from build123d import *

# Parameters (mm, degrees)
SKETCH_1_W          = 20
SKETCH_1_H          = 20
EXTRUDE_1_DEPTH     = 145
SKETCH_2_R          = 2.75
CUT_EXTRUDE_1_DEPTH = 20
SKETCH_4_R          = 1.5
CUT_EXTRUDE_4_DEPTH = 20


with BuildPart() as part:
    # 草图1 → 凸台-拉伸1 (new body)
    with BuildSketch(Plane.XY):
        Rectangle(SKETCH_1_W, SKETCH_1_H)
    extrude(amount=EXTRUDE_1_DEPTH)

    # 草图2 → 切除-拉伸1 (cut)
    with BuildSketch(Plane(origin=(10, 0, 0), x_dir=(0, 0, -1), z_dir=(1, 0, 0))):
        with Locations((-136, 3)):
            Circle(SKETCH_2_R)
        with Locations((-104, 3)):
            Circle(SKETCH_2_R)
        with Locations((-9, 3)):
            Circle(SKETCH_2_R)
        with Locations((-41, 3)):
            Circle(SKETCH_2_R)
    extrude(amount=-CUT_EXTRUDE_1_DEPTH, mode=Mode.SUBTRACT)

    # 草图4 → 切除-拉伸4 (cut)
    with BuildSketch(Plane(origin=(0, 10, 0), x_dir=(1, 0, 0), z_dir=(0, 1, 0))):
        with Locations(Location((-4.85, -24.606973042, 0), (0, 0, 270))):
            Circle(SKETCH_4_R)
        with Locations(Location((-4.85, -56.606973042, 0), (0, 0, 270))):
            Circle(SKETCH_4_R)
        with Locations(Location((-4.85, -72.606973042, 0), (0, 0, 270))):
            Circle(SKETCH_4_R)
        with Locations(Location((-4.85, -88.606973042, 0), (0, 0, 270))):
            Circle(SKETCH_4_R)
        with Locations(Location((-4.85, -120.606973042, 0), (0, 0, 270))):
            Circle(SKETCH_4_R)
        with Locations(Location((4.85, -120.606973042, 0), (0, 0, 270))):
            Circle(SKETCH_4_R)
        with Locations(Location((4.85, -88.606973042, 0), (0, 0, 270))):
            Circle(SKETCH_4_R)
        with Locations(Location((4.85, -72.606973042, 0), (0, 0, 270))):
            Circle(SKETCH_4_R)
        with Locations(Location((4.85, -56.606973042, 0), (0, 0, 270))):
            Circle(SKETCH_4_R)
        with Locations(Location((4.85, -24.606973042, 0), (0, 0, 270))):
            Circle(SKETCH_4_R)
    extrude(amount=-CUT_EXTRUDE_4_DEPTH, mode=Mode.SUBTRACT)


solid = part.part
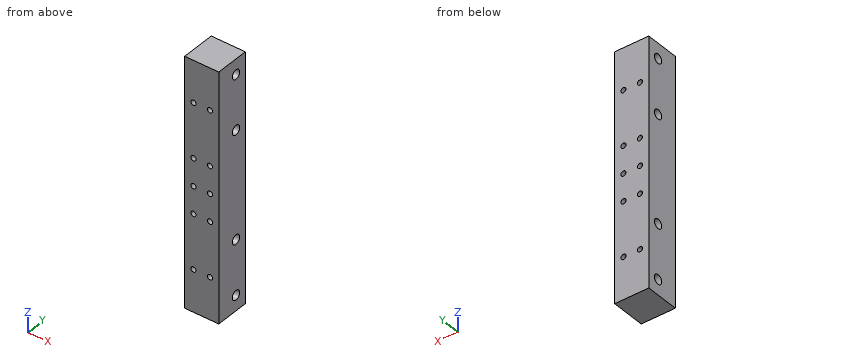
Part model, mm, in its own coordinate system. Give positions to 0.01 mm unless a question says otherwise; leave off trailing zeros. Write each loop counter-clockwise with the first axis right and the second up, starting at its lowest first coordinate (ties: lowest second). Pieces come first, ordered by that corner, then holes.
1) Pin check, flat tips, straight feed: pin 1 (2.5 mm diameter, centred on x = -4.85, z = 120.61, fed in from +Y); pin 2 (9 mm diameter, centred on y = 3, z = 9, fed in from -X). Stop position of each tip, or through.
Resolved:
pin 1: passes through
pin 2: stops at x = -10
2) Cut at A-A on x = 4.85. State how many separate pieces and enclosed holes the cut face has, then the cut area to 3 significant figures.
Resolved:
separate pieces: 6
enclosed holes: 4
area: 2,500 mm2
3) Cut at C-C on z = 136. Write the cut outline in (x, y).
Resolved:
outline: (-10, -10) - (10, -10) - (10, 0.25) - (-10, 0.25) - close; (-10, 5.75) - (10, 5.75) - (10, 10) - (-10, 10) - close
4) Cut at D-D on x = -1. Write the cut outline in (y, z).
Resolved:
outline: (-10, 0) - (10, 0) - (10, 145) - (-10, 145) - close; hole circle Ø5.5 at (3, 9); hole circle Ø5.5 at (3, 41); hole circle Ø5.5 at (3, 104); hole circle Ø5.5 at (3, 136)
5) Probe L1, parallel to Z at x = 5.5, y = -7.75; L2, parallel to Y at x = 4.25, z = 136; L3, parallel to Y at x = -9, z = 43. List the from-to ranges inside material, lowest first.
Resolved:
L1: z = 0 to 23.26, 25.96 to 55.26, 57.96 to 71.26, 73.96 to 87.26, 89.96 to 119.26, 121.96 to 145
L2: y = -10 to 0.25, 5.75 to 10
L3: y = -10 to 1.11, 4.89 to 10
